Source: CAD feature listing. Evaluate the final solid. Frame: model axes, mm. Give positions to 0.01 mm unless a question says otherwise; leave off trailing zeros. Write each loop counter-clockwise with the first axis right and the second up, starting at its lowest first coordinate (ties: lowest second). Pieces come first, ordered by that corner, then holes. Notation, with made-up numbers: M 67,79.25 L 75,79.25 A17 ccw 75,112.25 Z; hole C 37,3.25 d11. An arc over 180 degrees is marked long. Answer as a JSON object with one key per item and string values. Group by question number.
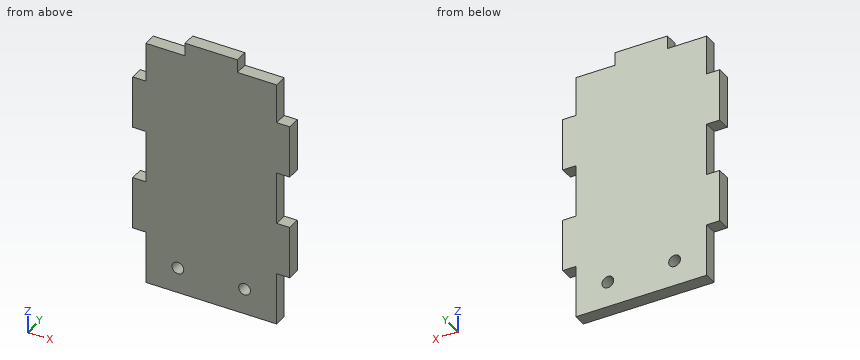
```python
from build123d import *

# Parameters (mm, degrees)
F0_R     = 2.25
F1_DEPTH = 5


with BuildPart() as f1:
    # F0 (on Front) → F1 (new body)
    with BuildSketch(Plane.XZ):
        Polygon((25, 32.5), (25, 47.5), (10, 47.5), (10, 52.5), (-10, 52.5), (-10, 47.5), (-25, 47.5), (-25, 32.5), (-30, 32.5), (-30, 12.5), (-25, 12.5), (-25, -7.5), (-30, -7.5), (-30, -27.5), (-25, -27.5), (-25, -47.5), (25, -47.5), (25, -27.5), (30, -27.5), (30, -7.5), (25, -7.5), (25, 12.5), (30, 12.5), (30, 32.5), align=None)
        with Locations((-12.75, -37.75)):
            Circle(F0_R, mode=Mode.SUBTRACT)
        with Locations((12.75, -37.75)):
            Circle(F0_R, mode=Mode.SUBTRACT)
    extrude(amount=F1_DEPTH)


solid = f1.part
```
(1) Section A-A, the plane x = -12.75. Return loops of the section in (y, z), plus the area to 4 significant figures.
(2) Section C-C, the plane y = -3.35. Return loops of the section in (x, z), plus the area to 3 significant figures.
(3) Ray query, L1, parallel to Z at x = 12.75, y = -1.35; L2, parallel to X at y = -4.5, z = -32.5; L3, parallel to Z at x = -16, y = -4.65. Return the intervals inside material, ascending. Write a range as [from, to].
(4) Section D-D, the plane z = 0. Return loops of the section in (x, y), plus the area to 3 significant figures.
(5) Section B-B, the plane z = -37.75. Return loops of the section in (x, y).
(6) Contact query for flat-ended pins moving along their axis: pin 1 Ø2 at (y, z) = (-2.5, 6.5) entering from +X; pin 2 Ø1.5 at (x, y) = (17.5, -1.5) entering from +Z; pin 3 Ø2.5 at (y, z) = (-3.5, 49.5) entering from -X. Output: stop coordinate, or through.
Reported:
{
 "1": {"outline": "M -5,-47.5 L 0,-47.5 L 0,-40 L -5,-40 Z; M -5,-35.5 L 0,-35.5 L 0,47.5 L -5,47.5 Z", "area": "452.5 mm2"},
 "2": {"outline": "M -30,-27.5 L -25,-27.5 L -25,-47.5 L 25,-47.5 L 25,-27.5 L 30,-27.5 L 30,-7.5 L 25,-7.5 L 25,12.5 L 30,12.5 L 30,32.5 L 25,32.5 L 25,47.5 L 10,47.5 L 10,52.5 L -10,52.5 L -10,47.5 L -25,47.5 L -25,32.5 L -30,32.5 L -30,12.5 L -25,12.5 L -25,-7.5 L -30,-7.5 Z; hole C -12.75,-37.75 d4.5; hole C 12.75,-37.75 d4.5", "area": "5,220 mm2"},
 "3": {"L1": "z = [-47.5, -40], [-35.5, 47.5]", "L2": "x = [-25, 25]", "L3": "z = [-47.5, 47.5]"},
 "4": {"outline": "M -25,-5 L 25,-5 L 25,0 L -25,0 Z", "area": "250 mm2"},
 "5": {"outline": "M -25,-5 L -15,-5 L -15,0 L -25,0 Z; M -10.5,-5 L 10.5,-5 L 10.5,0 L -10.5,0 Z; M 15,-5 L 25,-5 L 25,0 L 15,0 Z"},
 "6": {"pin 1": "stops at x = 25", "pin 2": "stops at z = 47.5", "pin 3": "stops at x = -10"}
}
